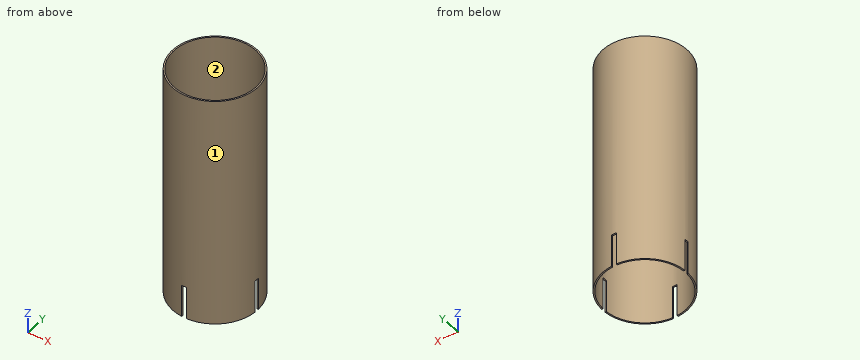
```python
from build123d import *

# Parameters (mm, degrees)
F0_R     = 9.05
F0_R_2   = 8.75
F1_DEPTH = 50
F2_W     = 1
F2_H     = 9.05
F3_DEPTH = 7
F4_COUNT = 2
F4_ANGLE = 90


with BuildPart() as f1:
    # F0 (on Top) → F1 (new body)
    with BuildSketch(Plane.XY):
        Circle(F0_R)
        Circle(F0_R_2, mode=Mode.SUBTRACT)
    extrude(amount=F1_DEPTH)


with BuildPart() as f3:
    # F2 (on Top) → F3 (new body)
    with BuildSketch(Plane.XY):
        with Locations((0, 4.525)):
            Rectangle(F2_W, F2_H)
        with Locations((0, -4.525)):
            Rectangle(F2_W, F2_H)
    extrude(amount=F3_DEPTH)


with BuildPart() as f4_1:
    # F4: instance of F3
    add(f3.part.rotate(Axis((0, 0, 0), (0, 0, -1)), 1 * F4_ANGLE / (F4_COUNT - 1)))


with BuildPart() as f1_1:
    add(f1.part)

    # F5: cut F3, F4_1
    add(f3.part, mode=Mode.SUBTRACT)
    add(f4_1.part, mode=Mode.SUBTRACT)


solid = f1_1.part
```
Part model, mm, in its own coordinate system. Face numbers are marked on the shaded views. Coordinates: 2 decimals unless noted, no trailing zeros. Loops run counter-clockwise (first coordinate to the right, second up) from the corner with the lowest first, then second, coordinate; pieces in that order, holes last. Notation, with made-up numbers: (81.25, 11.25) - (95.25, 11.25) arc R36 ccw to (95.25, 46.25) - close; hole circle Ø7 at (62, -38.75). An arc over 180 degrees is marked (long way). Write item = value, one per line. Start each with the question number.
Item 1: Cut at B-B, the plane x = -1. Give the cut face in (y, z), and give its area (3 significant figures).
Item 2: Flat gauge pins, fed straight in: pin 1 Ø1 at (x, z) = (-1, 16) entering from -Y; pin 2 Ø5 at (x, z) = (2, 20.5) entering from +Y; pin 3 Ø5 at (y, z) = (-6, 19) entering from -X. Where does each tip first touch, or does it go through?
Item 3: Mould opens along X. For the marked faces 1 and 2 say: released by +X, released by -X, zero draft, split by the parting line, or undercut.
Item 4: Cut at A-A, the plane y = 0. Give the cut face in (x, z), and give its area (3 significant figures).
Item 5: Wall check: L1, parallel to Y at x = 0, z = 38; L2, parallel to X at y = 0.5, z = 46; L3, parallel to X at y = -4.25, z = 37. Give the ranges that are in metal, low to high. Write a range as from..to.
Item 6: Cut at C-C, the plane z = 12.5. Give the cut face in (x, y).
The answers:
q1.outline = (-8.99, 0) - (-8.69, 0) - (-8.69, 50) - (-8.99, 50) - close; (8.69, 0) - (8.99, 0) - (8.99, 50) - (8.69, 50) - close
q1.area = 30.2 mm2
q2.pin_1 = -9.04
q2.pin_2 = 9.05
q2.pin_3 = -8.35
q3.face_1 = split by the parting line
q3.face_2 = undercut
q4.outline = (-9.05, 7) - (-8.75, 7) - (-8.75, 50) - (-9.05, 50) - close; (8.75, 7) - (9.05, 7) - (9.05, 50) - (8.75, 50) - close
q4.area = 25.8 mm2
q5.L1 = -9.05..-8.75, 8.75..9.05
q5.L2 = -9.04..-8.74, 8.74..9.04
q5.L3 = -7.99..-7.65, 7.65..7.99
q6.outline = circle Ø18.1 at (0, 0); hole circle Ø17.5 at (0, 0)
